Build history of the part. All positions in model axes, mm. A direction names the side the tool comes from. Give positions to 0.01 mm unless a question says otherwise; leave off trailing zeros. Write each loop counter-clockwise with the first axis right and the second up, starting at its lowest first coordinate (ties: lowest second). Pieces come first, ordered by that corner, then holes. Notation, with made-up numbers: (-5.75, 8) -> (12.25, 8) arc R30 cw to (12.25, 39) -> close; hole circle Ø2 at (38, 39.25). An arc over 180 degrees is marked (long way). Write item = value, one per line. Start each with the question number.
Q1. Mould opens along Z. For faces 5 (the face through (68, 48, -16)), 6 (the face through (10, 22, -48)), 7 (the face through (20, -15, 46)), 8 (the face through (15, 25, 46)) say: pulls with the +Z half, pulls with the -Z half, needs draft (parallel to the pull), parting line crosses it, or undercut.
Q2. Saw through at A-A, the plane z = -48. List the corners of the cut face in (x, y).
Q3. Saw through at C-C, the plane y = 35. List the corners of the cut face in (x, z).
Q4. Saw through at D-D, the plane x = 53. List the corners of the cut face in (y, z), then the cut area to 3 significant figures.
Q5. Drop flat-ended pins along their axis: P1, Ø9.5, axis at y = 59, z = -5, coming from the -X side; P2, Ø8, axis at x = 15.5, y = -12.5, coming from the +Z side; P3, Ø6.5, axis at x = 39, z = 48, coming from the +Y side. Give the stop position or say it passes through.
Q6. Saw through at B-B, the plane x = 34. List the corners of the cut face in (y, z).
Q7. Tool access for faces 1 (the face through (10, -21, 48)), 2 (the face through (15, 0, -50)), 3 (the face through (45, 46, 0)), 4 (the face through (20, -15, 52)): list every direction of +Z, -Z, +X, -X, +Y, -Y with a clear straight run to the whole face (end or side of a thin tool).
Q8. Wall check: line 1 (Z direction, x = 13, y = -3); line 2 (Z direction, x = 35, y = -3); line 3 (Y direction, x = 43, z = -7). Give the ranges that are in metal, low to high.
from build123d import *

# Parameters (mm, degrees)
EXTRUDE_1_DEPTH     = 20
SKETCH_2_W          = 4
SKETCH_2_H          = 30
EXTRUDE_3_DEPTH     = 20
SKETCH_4_R          = 60
SKETCH_4_R_2        = 50
CUT_EXTRUDE_2_DEPTH = 10
SKETCH_5_W          = 32
SKETCH_5_H          = 20
EXTRUDE_4_DEPTH     = 60
SKETCH_7_R          = 10
EXTRUDE_5_DEPTH     = 80
SKETCH_9_W          = 60
SKETCH_9_H          = 4
EXTRUDE_6_DEPTH     = 30
SKETCH_10_R         = 3
CUT_EXTRUDE_4_DEPTH = 135


with BuildPart() as part:
    # 草图1 → 凸台-拉伸1 (new body)
    with BuildSketch(Plane(origin=(0, 0, 0), x_dir=(0, 0, -1), z_dir=(1, 0, 0))):
        with BuildLine():
            Line((-50, 30), (-46, 30))
            Line((-46, 30), (-46, 19.595917942))
            ThreePointArc((-46, 19.595917942), (0, 50), (46, 19.595917942))
            Line((46, 19.595917942), (46, 30))
            Line((46, 30), (50, 30))
            Line((50, 30), (50, -30))
            Line((50, -30), (46, -30))
            Line((46, -30), (46, 0))
            ThreePointArc((46, 0), (0, 46), (-46, 0))
            Line((-46, 0), (-46, -30))
            Line((-46, -30), (-50, -30))
            Line((-50, -30), (-50, 30))
        make_face()
    extrude(amount=EXTRUDE_1_DEPTH)

    # 草图2 → 凸台-拉伸3 (add)
    with BuildSketch(Plane(origin=(20, 0, 0), x_dir=(0, 0, -1), z_dir=(1, 0, 0))):
        with Locations((-48, -15)):
            Rectangle(SKETCH_2_W, SKETCH_2_H)
        with Locations((48, -15)):
            Rectangle(SKETCH_2_W, SKETCH_2_H)
    extrude(amount=EXTRUDE_3_DEPTH)

    # 草图4 → 切除-拉伸2 (cut)
    with BuildSketch(Plane.ZY):
        Circle(SKETCH_4_R)
        Circle(SKETCH_4_R_2, mode=Mode.SUBTRACT)
    extrude(amount=-CUT_EXTRUDE_2_DEPTH, mode=Mode.SUBTRACT)

    # 草图5 → 凸台-拉伸4 (add)
    with BuildSketch(Plane.ZY.offset(-10)):
        with Locations((0, 56)):
            Rectangle(SKETCH_5_W, SKETCH_5_H)
    extrude(amount=-EXTRUDE_4_DEPTH)

    # 草图7 → 凸台-拉伸5 (add, symmetric)
    with BuildSketch(Plane.XY):
        with Locations((60, 56)):
            Circle(SKETCH_7_R)
    extrude(amount=EXTRUDE_5_DEPTH, both=True)

    # 草图9 → 凸台-拉伸6 (add)
    with BuildSketch(Plane.XZ.offset(30)):
        with Locations((50, -52)):
            Rectangle(SKETCH_9_W, SKETCH_9_H)
        with Locations((50, 52)):
            Rectangle(SKETCH_9_W, SKETCH_9_H)
    extrude(amount=-EXTRUDE_6_DEPTH)

    # 草图10 → 切除-拉伸4 (cut, through all)
    with BuildSketch(Plane.XY.offset(54)):
        with Locations((70, -15)):
            Circle(SKETCH_10_R)
    extrude(amount=-CUT_EXTRUDE_4_DEPTH, mode=Mode.SUBTRACT)


solid = part.part
Report:
q1.face_5 = pulls with the -Z half
q1.face_6 = needs draft
q1.face_7 = undercut
q1.face_8 = undercut
q2.outline = (0, -14) -> (10, -14) -> (10, -30) -> (40, -30) -> (40, 0) -> (20, 0) -> (20, 30) -> (10, 30) -> (10, 14) -> (0, 14) -> close; circle Ø20 at (60, 56)
q3.outline = (0, -35.71) -> (20, -35.71) -> (20, -29.85) -> (0, -29.85) -> close; (0, 29.85) -> (20, 29.85) -> (20, 35.71) -> (0, 35.71) -> close
q4.outline = (-30, -54) -> (0, -54) -> (0, -50) -> (-30, -50) -> close; (-30, 50) -> (0, 50) -> (0, 54) -> (-30, 54) -> close; (46, -16) -> (48.86, -16) -> (48.86, -80) -> (63.14, -80) -> (63.14, -16) -> (66, -16) -> (66, 16) -> (63.14, 16) -> (63.14, 80) -> (48.86, 80) -> (48.86, 16) -> (46, 16) -> close
q4.area = 2,710 mm2
q5.P1 = 10
q5.P2 = 50
q5.P3 = 0
q6.outline = (-30, -54) -> (0, -54) -> (0, -46) -> (-30, -46) -> close; (-30, 46) -> (0, 46) -> (0, 54) -> (-30, 54) -> close; (46, -16) -> (66, -16) -> (66, 16) -> (46, 16) -> close
q7.face_1 = +Z, -X, -Y
q7.face_2 = -Z, -X, +Y, -Y
q7.face_3 = +Z, -Z, +X, -Y
q7.face_4 = +Z, -X, +Y, -Y
q8.line_1 = -50 to -46, 46 to 50
q8.line_2 = -54 to -46, 46 to 54
q8.line_3 = 46 to 66
